The listing builds one solid part. Answer for the finished solid, in the listing's coordinates (mm). Face numbers are marked on the shaded views. A direction names the side the tool comes from. Round coordinates to 2 decimals unless told otherwise and drop trailing zeros. Loops run counter-clockwise (first coordinate to the right, second up) from the corner with the lowest first, then second, coordinate; pieces in that order, holes last. Notation, with made-up numbers: (-34, -21.5) -> (2, -21.5) arc R20 ccw to (2, -10.5) -> close; hole circle Ø6 at (41, 30.5). An arc over 180 degrees is marked (long way). Answer in a Markdown table with one row per item. Add a question column.
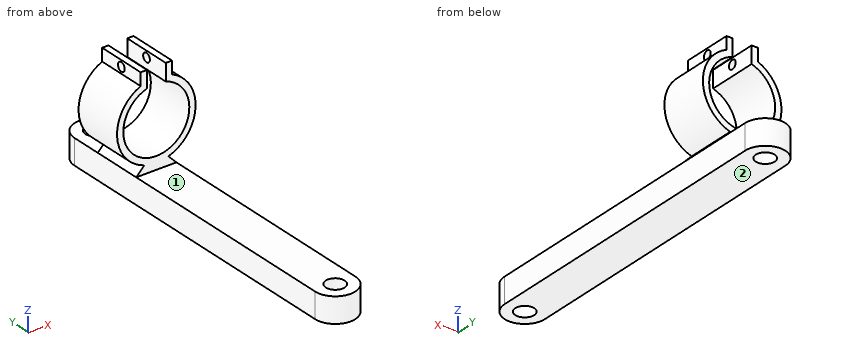
```python
from build123d import *

# Parameters (mm, degrees)
SKETCH1_R           = 1.905
BOSS_EXTRUDE1_DEPTH = 5.08
BOSS_EXTRUDE2_START = 10.16
BOSS_EXTRUDE2_DEPTH = 10.16
SKETCH3_R           = 0.889
CUT_EXTRUDE1_DEPTH  = 12.1125


with BuildPart() as part:
    # Sketch1 → Boss-Extrude1 (new body)
    with BuildSketch(Plane(origin=(-856.488519717, 635.703940982, 371.824950285), x_dir=(1, 0, 0), z_dir=(0, 0, 1))):
        with BuildLine():
            Line((4.064, 31.75), (4.064, -31.75))
            ThreePointArc((4.064, -31.75), (0, -35.814), (-4.064, -31.75))
            Line((-4.064, -31.75), (-4.064, 31.75))
            ThreePointArc((-4.064, 31.75), (0, 35.814), (4.064, 31.75))
        make_face()
        with Locations((0, -31.75)):
            Circle(SKETCH1_R, mode=Mode.SUBTRACT)
        with Locations((0, 31.75)):
            Circle(SKETCH1_R, mode=Mode.SUBTRACT)
    extrude(amount=BOSS_EXTRUDE1_DEPTH)

    # Sketch2 → Boss-Extrude2 (add)
    with BuildSketch(Plane.XZ.offset(-671.517940982).offset(BOSS_EXTRUDE2_START)):
        with BuildLine():
            Line((-854.05175925, 378.554950285), (-852.424519717, 376.904950285))
            Line((-852.424519717, 376.904950285), (-860.552519717, 376.904950285))
            Line((-860.552519717, 376.904950285), (-858.925280183, 378.554950285))
            ThreePointArc((-858.925280183, 378.554950285), (-864.416201891, 385.714494899), (-859.663519717, 393.384000256))
            Line((-859.663519717, 393.384000256), (-859.663519717, 395.924000256))
            Line((-859.663519717, 395.924000256), (-858.393519717, 395.924000256))
            Line((-858.393519717, 395.924000256), (-858.393519717, 393.814671139))
            Line((-858.393519717, 393.814671139), (-858.393519717, 392.498725586))
            ThreePointArc((-858.393519717, 392.498725586), (-856.488519717, 379.441661341), (-854.583519717, 392.498725586))
            Line((-854.583519717, 392.498725586), (-854.583519717, 393.814671139))
            Line((-854.583519717, 393.814671139), (-854.583519717, 395.924000256))
            Line((-854.583519717, 395.924000256), (-853.313519717, 395.924000256))
            Line((-853.313519717, 395.924000256), (-853.313519717, 393.384000256))
            ThreePointArc((-853.313519717, 393.384000256), (-848.560837543, 385.714494899), (-854.05175925, 378.554950285))
        make_face()
    extrude(amount=BOSS_EXTRUDE2_DEPTH)

    # Sketch3 → Cut-Extrude1 (cut, through all)
    with BuildSketch(Plane(origin=(-853.313519717, 0, 0), x_dir=(0, 0, -1), z_dir=(1, 0, 0))):
        with Locations((-394.654000256, 656.277940982)):
            Circle(SKETCH3_R)
    extrude(amount=-CUT_EXTRUDE1_DEPTH, mode=Mode.SUBTRACT)


solid = part.part
```
Item 1: Flat-ended cylindrical pins translate along their axes: P1, Ø1.5, axis at x = -862, z = 383, coming from the -Y side; P2, Ø6.5, axis at x = -856, y = 667, coming from the +Z side; P3, Ø1, axis at x = -856, y = 659, coming from the +Z side; P4, Ø10, axis at y = 663, z = 385, coming from the -X side. Find the tip coordinate at first contact, or state that the pin passes through.
Item 2: Section B-B, the plane x = -851 is taken. Write down the section's boundary in (y, z), and give its area (3 significant figures).
Item 3: Section A-A, the plane z = 383.75 is taken. Write down the section's boundary in (x, y), and give its area (3 significant figures).
Item 4: For the marked faces 1 and 2, determine the directions among +Z, -Z, +X, -X, +Y, -Y from which every point of the face is accessible in a straight line to the end or side of a thin tool.
Item 5: Section D-D, the plane x = -856.25 is taken. Write down the section's boundary in (y, z), and give its area (3 significant figures).
Item 6: Consider L1, parallel to Z at x = -859.5, y = 637.5; L2, parallel to Y at x = -849.5, z = 384.25; L3, parallel to X at y = 651, z = 373.5. Determine where each line is inside the solid, lowest interval first. Write a range as from..to.
Item 7: Section C-C, the plane z = 394.75 is taken. Write down the section's boundary in (x, y).
Here are the results:
| question | item | result |
|---|---|---|
| 1 | P1 | stops at y = 651.2 |
| 1 | P2 | stops at z = 376.9 |
| 1 | P3 | stops at z = 379.52 |
| 1 | P4 | stops at x = -864.43 |
| 2 | outline | (651.2, 380.38) -> (661.36, 380.38) -> (661.36, 382.32) -> (651.2, 382.32) -> close; (651.2, 389.89) -> (661.36, 389.89) -> (661.36, 391.84) -> (651.2, 391.84) -> close |
| 2 | area | 39.6 mm² |
| 3 | outline | (-864.07, 651.2) -> (-862.72, 651.2) -> (-862.72, 661.36) -> (-864.07, 661.36) -> close; (-850.25, 651.2) -> (-848.91, 651.2) -> (-848.91, 661.36) -> (-850.25, 661.36) -> close |
| 3 | area | 27.3 mm² |
| 4 | face 1 | +Z, +X, -X, -Y |
| 4 | face 2 | -Z, +X, -X, +Y, -Y |
| 5 | outline | (599.9, 371.82) -> (602.06, 371.82) -> (602.06, 376.9) -> (599.9, 376.9) -> close; (605.84, 371.82) -> (665.56, 371.82) -> (665.56, 376.9) -> (661.36, 376.9) -> (661.36, 379.45) -> (651.2, 379.45) -> (651.2, 376.9) -> (605.84, 376.9) -> close; (669.34, 371.82) -> (671.51, 371.82) -> (671.51, 376.9) -> (669.34, 376.9) -> close |
| 5 | area | 351 mm² |
| 6 | L1 | z = 371.82..376.9 |
| 6 | L2 | y = 651.2..661.36 |
| 6 | L3 | x = -860.55..-852.42 |
| 7 | outline | (-859.66, 651.2) -> (-858.39, 651.2) -> (-858.39, 655.39) -> (-859.66, 655.39) -> close; (-859.66, 657.16) -> (-858.39, 657.16) -> (-858.39, 661.36) -> (-859.66, 661.36) -> close; (-854.58, 651.2) -> (-853.31, 651.2) -> (-853.31, 655.39) -> (-854.58, 655.39) -> close; (-854.58, 657.16) -> (-853.31, 657.16) -> (-853.31, 661.36) -> (-854.58, 661.36) -> close |
